```python
from build123d import *

# Parameters (mm, degrees)
SKETCH1_W             = 15
SKETCH1_H             = 60
BOSS_EXTRUDE1_DEPTH   = 1
BOSS_EXTRUDE1_2_DEPTH = 1
SKETCH1_3_W           = 10
SKETCH1_3_H           = 60
BOSS_EXTRUDE2_DEPTH   = 3
CUT_EXTRUDE1_DEPTH    = 66
SKETCH5_R             = 1
CUT_EXTRUDE2_DEPTH    = 10


with BuildPart() as part:
    # Sketch1 → Boss-Extrude1 (new body)
    with BuildSketch(Plane(origin=(0, 0, 0), x_dir=(0, 1, 0), z_dir=(0, 0, 1))):
        with Locations((-12.5, 0)):
            Rectangle(SKETCH1_W, SKETCH1_H)
    extrude(amount=BOSS_EXTRUDE1_DEPTH)



with BuildPart() as body_2:
    # Sketch1 → Boss-Extrude1 2 (new body)
    with BuildSketch(Plane(origin=(0, 0, 0), x_dir=(0, 1, 0), z_dir=(0, 0, 1))):
        with Locations((12.5, 0)):
            Rectangle(SKETCH1_W, SKETCH1_H)
    extrude(amount=BOSS_EXTRUDE1_2_DEPTH)


with BuildPart() as part_1:
    add(part.part)

    add(body_2.part)  # Boss-Extrude2 merges body 2
    # Sketch1<3> → Boss-Extrude2 (add)
    with BuildSketch(Plane(origin=(0, 0, 0), x_dir=(0, 1, 0), z_dir=(0, 0, 1))):
        Rectangle(SKETCH1_3_W, SKETCH1_3_H)
    extrude(amount=BOSS_EXTRUDE2_DEPTH)

    # Sketch2 → Cut-Extrude1 (cut)
    with BuildSketch(Plane.YZ.offset(30)):
        Polygon((-5, 1), (-4, 1), (-5, 3), align=None)
        Polygon((5, 1), (4, 1), (5, 3), align=None)
    extrude(amount=-CUT_EXTRUDE1_DEPTH, mode=Mode.SUBTRACT)

    # Sketch5 → Cut-Extrude2 (cut)
    with BuildSketch(Plane.XY.offset(3)):
        with Locations((-27.5, 0)):
            Circle(SKETCH5_R)
        with Locations((27.5, 0)):
            Circle(SKETCH5_R)
    extrude(amount=-CUT_EXTRUDE2_DEPTH, mode=Mode.SUBTRACT)


solid = part_1.part
```
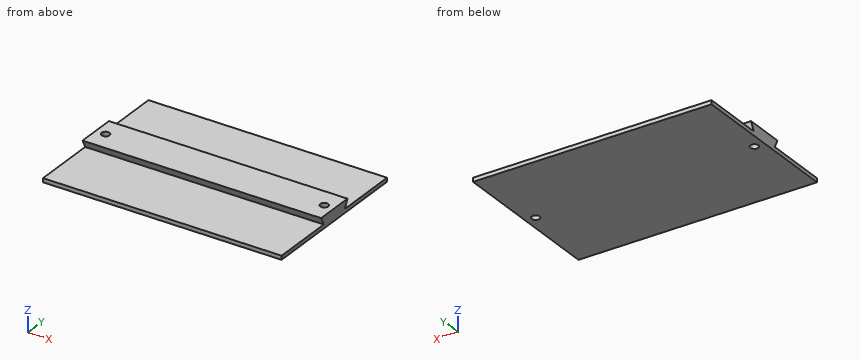
The model under review builds one solid part; all positions refer to its coordinate system, in mm. Give positions to 0.01 mm unless a question says otherwise; leave off trailing zeros. Write each loop counter-clockwise with the first axis right and the second up, starting at its lowest first coordinate (ties: lowest second). Pieces come first, ordered by that corner, then holes. Notation, with made-up numbers: M 48,63 L 54,63 A31 ccw 54,94 Z; hole C -26.5,56.5 d4. An arc over 180 degrees is marked long. Answer in a Markdown table with one row per item.
Item 1: Add section D-D on x = -11. Give the boundary of the cut face in (y, z).
Check sheet entries:
| item | result |
|---|---|
| outline | M -20,0 L 20,0 L 20,1 L 4,1 L 5,3 L -5,3 L -4,1 L -20,1 Z |
Item 2: Add section A-A on y = 0. Give the boundary of the cut face in (x, z), plus the area to 3 significant figures.
Check sheet entries:
| item | result |
|---|---|
| outline | M -30,0 L -28.5,0 L -28.5,3 L -30,3 Z; M -26.5,0 L 26.5,0 L 26.5,3 L -26.5,3 Z; M 28.5,0 L 30,0 L 30,3 L 28.5,3 Z |
| area | 168 mm2 |
Item 3: For P1, Ø17.5, axis at x = 11.5, y = 9.5, coming from the +Z side; P2, Ø8, axis at x = -11, y = -16, coming from the +Z side, all flat-tipped, find the tip position at first contact; note any pin that passes through.
Check sheet entries:
| item | result |
|---|---|
| P1 | z = 3 |
| P2 | z = 1 |
Item 4: Add section B-B on x = 27.5. Give the boundary of the cut face in (y, z).
Check sheet entries:
| item | result |
|---|---|
| outline | M -20,0 L -1,0 L -1,3 L -5,3 L -4,1 L -20,1 Z; M 1,0 L 20,0 L 20,1 L 4,1 L 5,3 L 1,3 Z |
Item 5: For line 1 along Z through (x, y) = (-10.5, -12); line 2 along Y through (x, z) = (27.5, 2); line 3 along Y through (x, z) = (27.5, 1.5), list the stretches that pass through material, from the lowest coordinate up.
Check sheet entries:
| item | result |
|---|---|
| line 1 | 0 to 1 |
| line 2 | -4.5 to -1, 1 to 4.5 |
| line 3 | -4.25 to -1, 1 to 4.25 |
Item 6: Add section C-C on z = 1.6. Give the boundary of the cut face in (x, y).
Check sheet entries:
| item | result |
|---|---|
| outline | M -30,-4.3 L 30,-4.3 L 30,4.3 L -30,4.3 Z; hole C -27.5,0 d2; hole C 27.5,0 d2 |
